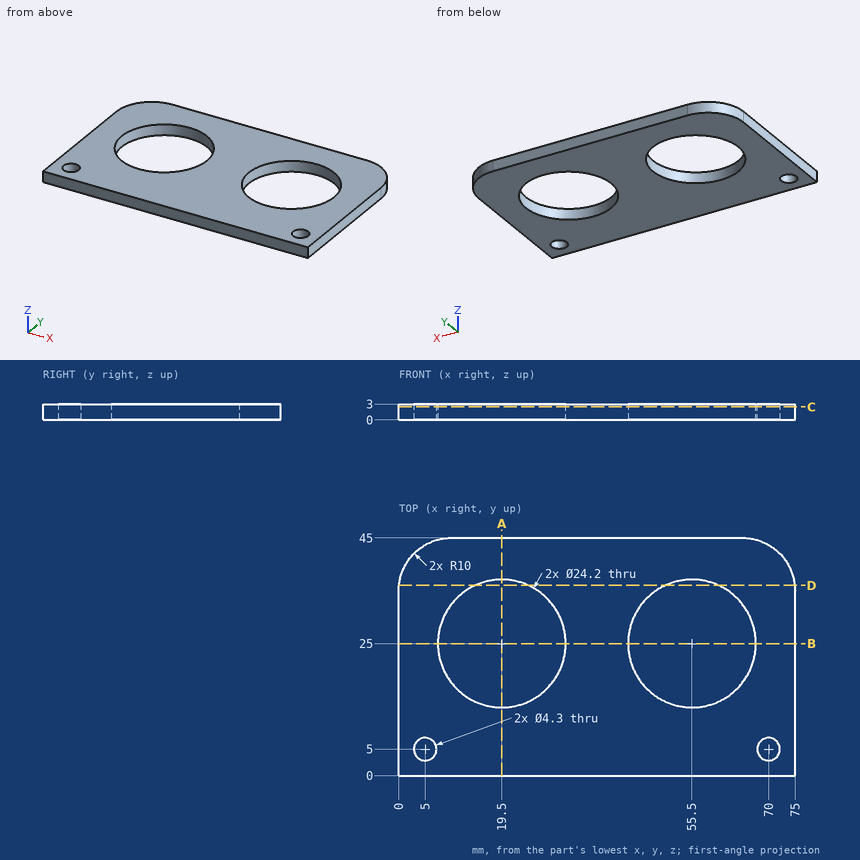
Here's the drawing with two shaded views (mm, measured from the low corner). I have some questions. Give positions to 0.01 mm unless a question says otherwise; leave off trailing zeros. Write each loop counter-clockwise with the first axis right and the second up, starting at its lowest first coordinate (ties: lowest second). Pieces come first, ordered by that corner, then holes. Notation, with made-up numbers: (1, -36) -> (19, -36) arc R36 ccw to (19, 1) -> close; hole circle Ø9 at (6.25, 67). An arc over 180 degrees is marked (long way). Use one line per item in the form item = value. Start each with the question number.
1. Imagine slicing it at A-A on x = 19.5. List the corners of the cut face in (y, z) for me, plus the area to 3 significant figures.
2. Imagine slicing it at C-C on z = 2.45. List the corners of the cut face in (x, y) for me.
3. Imagine slicing it at B-B on y = 25. List the corners of the cut face in (x, z) for me.
4. Imagine slicing it at D-D on y = 36. List the corners of the cut face in (x, z) for me.
5. If I drill on L1, parallel to X at y = 21.5, z = 1.7; L2, parallel to Y at x = 55.5, z = 2.15; L3, parallel to X at y = 33.5, z = 1.25, over which ranges is the centre line in solid material (lowest first)?
6. Will this pin go through, and if not, where does the flat tip stop? pin 1 Ø4 at (x, y) = (70, 5) entering from +Z.
Entries:
q1.outline = (0, 0) -> (12.9, 0) -> (12.9, 3) -> (0, 3) -> close; (37.1, 0) -> (45, 0) -> (45, 3) -> (37.1, 3) -> close
q1.area = 62.4 mm²
q2.outline = (0, 0) -> (75, 0) -> (75, 35) arc R10 ccw to (65, 45) -> (10, 45) arc R10 ccw to (0, 35) -> close; hole circle Ø4.3 at (5, 5); hole circle Ø24.2 at (19.5, 25); hole circle Ø24.2 at (55.5, 25); hole circle Ø4.3 at (70, 5)
q3.outline = (0, 0) -> (7.4, 0) -> (7.4, 3) -> (0, 3) -> close; (31.6, 0) -> (43.4, 0) -> (43.4, 3) -> (31.6, 3) -> close; (67.6, 0) -> (75, 0) -> (75, 3) -> (67.6, 3) -> close
q4.outline = (0.05, 0) -> (14.46, 0) -> (14.46, 3) -> (0.05, 3) -> close; (24.54, 0) -> (50.46, 0) -> (50.46, 3) -> (24.54, 3) -> close; (60.54, 0) -> (74.95, 0) -> (74.95, 3) -> (60.54, 3) -> close
q5.L1 = 0 to 7.92, 31.08 to 43.92, 67.08 to 75
q5.L2 = 0 to 12.9, 37.1 to 45
q5.L3 = 0 to 10.89, 28.11 to 46.89, 64.11 to 75
q6.pin_1 = through
